Geometry: final body of the model. Coordinates: model frame, mm. A direction names the side the tool comes from. Give positions to 0.01 mm unless a question says otherwise; leave off trailing zeros. Write each loop counter-clockwise with the first axis right and the second up, starting at its lowest first coordinate (ties: lowest second). Pieces come first, ordered by that corner, then holes.
Q1. Section D-D (x = -25.5). Return the cut outline in (y, z).
Q2. Section C-C (z = -5). Return the cut outline in (x, y).
Q3. Section B-B (y = 7). Return the cut outline in (x, z), plus the area to 3 significant figures.
Q4. Mould query, pull axis Y, two halves, no side actions, for faces 3 (the cylindrical face through (-50.904, 14.556, 1.982)), 4 (the cylindrical face through (8.024, 12.859, -86.462)), 5 (the flat face through (-51, 17.78, -39)), 6 (the cylindrical face through (-45.165, 2.504, 14.2)). Classes: +Y half, -Y half, draft (parallel to the pull), parting line (faces both ways), or undercut.
Q5. Line query: line 1 (X direction, y = 10.25, z = -16); line 2 (Y direction, x = 2, z = -12). Output: solid intervals per line, ascending.
Q6. Section A-A (y = 12.78). Return the cut outline in (x, z), plus the area to 3 significant figures.
Q7. Reachability of faces 1 (the flat face through (-48.65, 11, -37)), 2 (the cylindrical face through (8.024, 14.556, 1.982)) from +Z, -Z, +X, -X, +Y, -Y: full face, straight path, thin tool, end or side. Return the list, or none.
Q8. Pin query (flat end, axial travel): pin 1 Ø1 at (x, z) = (-38, -65.5) entering from +Y; pin 2 Ø3 at (y, z) = (12.78, -88.25) entering from -X. Return the tip coordinate at first contact, or that it passes through.
from build123d import *

# Parameters (mm, degrees)
SKETCH2_W           = 63.5
SKETCH2_H           = 120
BOSS_EXTRUDE1_DEPTH = 5.08
SKETCH3_W           = 4.572
SKETCH3_H           = 120
BOSS_EXTRUDE2_DEPTH = 12.7
CUT_EXTRUDE1_REACH  = 120.329
SKETCH4_R           = 1.79097934
SKETCH5_R           = 1.75
CUT_EXTRUDE2_DEPTH  = 114.146112049


with BuildPart() as part:
    # Sketch2 → Boss-Extrude1 (new body)
    with BuildSketch(Plane(origin=(0, 0, 0), x_dir=(1, 0, 0), z_dir=(0, 1, 0))):
        with Locations((-21.471987722, 38.251383169)):
            Rectangle(SKETCH2_W, SKETCH2_H)
    extrude(amount=BOSS_EXTRUDE1_DEPTH)

    # Sketch3 → Boss-Extrude2 (add)
    with BuildSketch(Plane(origin=(0, 5.08, 0), x_dir=(1, 0, 0), z_dir=(0, 1, 0))):
        with Locations((-50.935987722, 38.251383169)):
            Rectangle(SKETCH3_W, SKETCH3_H)
        with Locations((7.992012278, 38.251383169)):
            Rectangle(SKETCH3_W, SKETCH3_H)
    extrude(amount=BOSS_EXTRUDE2_DEPTH)

    # Cut-Extrude1: up to this face of the body (flat: up to its plane)
    cut_extrude1_end = Plane(part.part.faces().sort_by_distance((-53.221987722, 8.89, -38.251383169))[0])
    # Sketch4 → Cut-Extrude1 (cut, up to the picked face)
    with BuildSketch(Plane(origin=(10.278012278, 0, 0), x_dir=(0, 0, -1), z_dir=(1, 0, 0)), mode=Mode.PRIVATE) as cut_extrude1_sk1:
        with Locations((-1.748616831, 12.78)):
            Circle(SKETCH4_R)
    cut_extrude1_tool1 = split(extrude(cut_extrude1_sk1.sketch, amount=-CUT_EXTRUDE1_REACH, mode=Mode.PRIVATE), bisect_by=cut_extrude1_end, keep=Keep.BOTH, mode=Mode.PRIVATE)
    # Sketch4 → Cut-Extrude1 (cut, up to the picked face)
    with BuildSketch(Plane(origin=(10.278012278, 0, 0), x_dir=(0, 0, -1), z_dir=(1, 0, 0)), mode=Mode.PRIVATE) as cut_extrude1_sk2:
        with Locations((88.251383169, 12.78)):
            Circle(SKETCH4_R)
    cut_extrude1_tool2 = split(extrude(cut_extrude1_sk2.sketch, amount=-CUT_EXTRUDE1_REACH, mode=Mode.PRIVATE), bisect_by=cut_extrude1_end, keep=Keep.BOTH, mode=Mode.PRIVATE)
    add(cut_extrude1_tool1.solids().sort_by(Axis((10.278012, 12.78, 1.748617), (-1, 0, 0)))[0], mode=Mode.SUBTRACT)
    add(cut_extrude1_tool2.solids().sort_by(Axis((10.278012, 12.78, -88.251383), (-1, 0, 0)))[0], mode=Mode.SUBTRACT)

    # Sketch5 → Cut-Extrude2 (cut, through all)
    with BuildSketch(Plane(origin=(0, 0, 0), x_dir=(-1, 0, 0), z_dir=(0, -1, 0))):
        with Locations(Location((43.456413511, 91.179295555, 0), (0, 0, 90))):
            Circle(SKETCH5_R)
        with Locations(Location((0.456413511, 91.179295555, 0), (0, 0, 90))):
            Circle(SKETCH5_R)
        with Locations(Location((43.456413511, -13.820704445, 0), (0, 0, 90))):
            Circle(SKETCH5_R)
        with Locations(Location((0.456413511, -13.820704445, 0), (0, 0, 90))):
            Circle(SKETCH5_R)
    extrude(amount=-CUT_EXTRUDE2_DEPTH, mode=Mode.SUBTRACT)


solid = part.part
Computed:
1. outline: (0, -98.25) - (5.08, -98.25) - (5.08, 21.75) - (0, 21.75) - close
2. outline: (-53.22, 0) - (10.28, 0) - (10.28, 17.78) - (5.71, 17.78) - (5.71, 5.08) - (-48.65, 5.08) - (-48.65, 17.78) - (-53.22, 17.78) - close
3. outline: (-53.22, -98.25) - (-48.65, -98.25) - (-48.65, 21.75) - (-53.22, 21.75) - close; (5.71, -98.25) - (10.28, -98.25) - (10.28, 21.75) - (5.71, 21.75) - close
3. area: 1,100 mm2
4. face 3: undercut
4. face 4: undercut
4. face 5: +Y half
4. face 6: draft
5. line 1: x = -53.22 to -48.65, 5.71 to 10.28
5. line 2: y = 0 to 5.08
6. outline: (-53.22, -98.25) - (-48.65, -98.25) - (-48.65, -90.04) - (-53.22, -90.04) - close; (-53.22, -86.46) - (-48.65, -86.46) - (-48.65, -0.04) - (-53.22, -0.04) - close; (-53.22, 3.54) - (-48.65, 3.54) - (-48.65, 21.75) - (-53.22, 21.75) - close; (5.71, -98.25) - (10.28, -98.25) - (10.28, -90.04) - (5.71, -90.04) - close; (5.71, -86.46) - (10.28, -86.46) - (10.28, -0.04) - (5.71, -0.04) - close; (5.71, 3.54) - (10.28, 3.54) - (10.28, 21.75) - (5.71, 21.75) - close
6. area: 1,030 mm2
7. face 1: +Z, -Z, +Y
7. face 2: +X, -X
8. pin 1: stops at y = 5.08
8. pin 2: passes through
